CAD build for the part. Positions are in the model's coordinates, mm. Round coordinates to 2 decimals unless told otherwise and drop trailing zeros. Write each loop counter-clockwise with the first axis right and the second up, starting at its lowest first coordinate (ties: lowest second). Pieces come first, ordered by that corner, then holes. Notation, with made-up numbers: (28.5, 68) - (40.5, 68) arc R23 cw to (40.5, 94) - close; hole circle Ø6 at (11, 38.5). An arc over 180 degrees is marked (long way). Put each result on its own line as item: value. Start each with the question number.
Item 1: Cut at B-B (y = -155). Give the cut face in (x, z).
Item 2: Pin check, flat tips, straight feed: pin 1 Ø1.5 at (y, z) = (-210, 1) entering from +X; pin 2 Ø3.5 at (x, y) = (75, -60) entering from +Z; pin 3 Ø0.9 at (x, z) = (-224, 2) entering from -Y. Stop position of each tip, or through.
Item 3: Drill centre lines: line 1 (Y direction, x = -75, z = 1.35); line 2 (Y direction, x = 0, z = 1.65); line 3 (X direction, y = 210.5, z = 0.6). Where is each one in solid material? Low to high. Write a range as from..to.
Item 4: Cut at A-A (z = 1.9). Give the cut face in (x, y).
Autodesk Inventor part; units mm, degrees
ref_plane "YZ Plane" through (0, 0, 0) normal (1, 0, 0) x (0, 1, 0)
ref_plane "XZ Plane" through (0, 0, 0) normal (0, 1, 0) x (-1, 0, 0)
ref_plane "XY Plane" through (0, 0, 0) normal (0, 0, 1) x (1, 0, 0)
sketch "Skizze1" plane through (0, 0, 0) normal (0, 0, 1) x (1, 0, 0)
  line L0 (-235, -235) -> (235, -235)
  line L1 (235, -235) -> (235, 235)
  line L2 (235, 235) -> (-235, 235)
  line L3 (-235, 235) -> (-235, -235)
  line L4 (-235, -235) -> (235, 235) construction
  line L5 (235, -235) -> (-235, 235) construction
  line L6 (-235, -235) -> (-215, -235)
  line L7 (-215, -235) -> (-215, -200)
  line L8 (-215, -200) -> (-235, -200)
  line L9 (-235, -200) -> (-235, -235)
  line L10 (235, -235) -> (215, -235)
  line L11 (215, -235) -> (215, -200)
  line L12 (215, -200) -> (235, -200)
  line L13 (235, -200) -> (235, -235)
  line L14 (235, 235) -> (215, 235)
  line L15 (215, 235) -> (215, 200)
  line L16 (215, 200) -> (235, 200)
  line L17 (235, 200) -> (235, 235)
  line L18 (-235, 235) -> (-215, 235)
  line L19 (-215, 235) -> (-215, 200)
  line L20 (-215, 200) -> (-235, 200)
  line L21 (-235, 200) -> (-235, 235)
  line L22 (-10, -235) -> (10, -235)
  line L23 (10, -235) -> (10, -215)
  line L24 (10, -215) -> (-10, -215)
  line L25 (-10, -215) -> (-10, -235)
  circle A0 centre (0, -155) radius 7.5
  circle A1 centre (-75, 60) radius 3
  circle A2 centre (75, 60) radius 3
  circle A3 centre (75, -60) radius 3
  circle A4 centre (-75, -60) radius 3
  line L26 (-75, -60) -> (75, -60) construction
  line L27 (75, -60) -> (75, 60) construction
  line L28 (75, 60) -> (-75, 60) construction
  line L29 (-75, 60) -> (-75, -60) construction
  line L30 (-75, -60) -> (75, 60) construction
  line L31 (75, -60) -> (-75, 60) construction
  point P0 (0, 0)
  point P1 (0, -235)
  dimension "d0" = 470
  dimension "d1" = 470
  dimension "d4" = 35
  dimension "d5" = 20
  dimension "d6" = 20
  dimension "d7" = 20
  dimension "d8" = 15
  dimension "d9" = 80
  dimension "d10" = 150
  dimension "d11" = 120
  dimension "d12" = 6
extrude "Extrusion1" add sketch "Skizze1" along normal blind 3 contours L7 L8 L3 L20 L19 L2 L15 L16 L1 L12 L11 L0 L23 L24 L25
properties part number "Panel Bottom" material "Polycarbonat, klar"
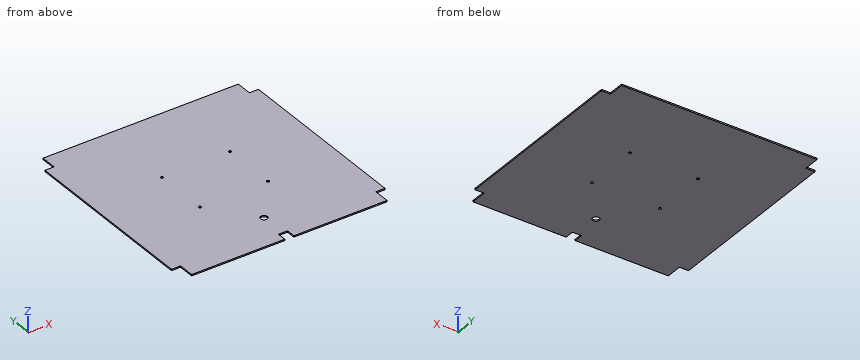
Output values:
1. outline: (-235, 0) - (-7.5, 0) - (-7.5, 3) - (-235, 3) - close; (7.5, 0) - (235, 0) - (235, 3) - (7.5, 3) - close
2. pin 1: x = 215
2. pin 2: through
2. pin 3: y = -200
3. line 1: -235..-63, -57..57, 63..235
3. line 2: -215..-162.5, -147.5..235
3. line 3: -215..215
4. outline: (-235, -200) - (-215, -200) - (-215, -235) - (-10, -235) - (-10, -215) - (10, -215) - (10, -235) - (215, -235) - (215, -200) - (235, -200) - (235, 200) - (215, 200) - (215, 235) - (-215, 235) - (-215, 200) - (-235, 200) - close; hole circle Ø6 at (-75, -60); hole circle Ø6 at (-75, 60); hole circle Ø15 at (0, -155); hole circle Ø6 at (75, -60); hole circle Ø6 at (75, 60)
